Source: CAD feature listing. Evaluate the final solid. Frame: model axes, mm. Face numbers are marked on the shaded views. A direction names the side the tool comes from. Give positions to 0.01 mm unless a question says otherwise; leave off trailing zeros. Order: outer loops, then holes, each group sorted by start corner. A loop starts at its lowest first (then second) coordinate and runs counter-clockwise, first axis right, second up.
1) Section C-C, the plane x = -15. Return loops of the section in (y, z), plus the area to 3 significant figures.
2) Section A-A, the plane y = 4.75. Return loops of the section in (x, z) (1 decimal).
3) Section B-B, the plane z = -11.07. Return loops of the section in (x, y) (3 decimals), plus the area to 3 significant figures.
4) Material intervals for line 1 (X direction, y = 2.25, z = 2.75) (1 decimal); line 2 (Z direction, x = -26, y = 2.25); line 3 (Y direction, x = 9.5, z = 6.25), sorted ascending.
5) Draft query along X for the marked faces 4, 5 and 6. Return one class per face: released by +X, released by -X, zero draft, split by the parting line, or undercut.
6) Access query for the marked faces 1, 2 and 3. Directions: +Z, -Z, +X, -X, +Y, -Y. A direction counts if a zero-diameter tool reaches every point of the face in a straight line with its end or side. Return the directions, or none.
7) Section D-D, the plane z = 6.5. Return loops of the section in (x, y) (1 decimal), plus the area to 3 significant figures.
8) First-contact query: P1, Ø1.9, axis at x = -15.5, z = 5.5, coming from the +Y side; P2, Ø2, axis at y = 3, z = 5, coming from the -X side; P3, Ø2, axis at y = 3, z = 4.5, coming from the +X side (3 decimals); P4, Ø4, axis at x = 27, y = 7.5, coming from the -Z side. Flat tips, straight axial feed; report the tip coordinate or a pass-through.
Autodesk Inventor part; units mm, degrees
ref_plane "YZ Plane" through (0, 0, 0) normal (1, 0, 0) x (0, 1, 0)
ref_plane "XZ Plane" through (0, 0, 0) normal (0, 1, 0) x (-1, 0, 0)
ref_plane "XY Plane" through (0, 0, 0) normal (0, 0, 1) x (1, 0, 0)
sketch "Sketch1" plane through (0, 0, 0) normal (0, 1, 0) x (-1, 0, 0)
  line L0 (36.775, 13.07) -> (-36.775, 13.07)
  line L1 (-36.775, 13.07) -> (-36.775, -13.07)
  line L2 (-36.775, -13.07) -> (36.775, -13.07)
  line L3 (36.775, -13.07) -> (36.775, 13.07)
  line L4 (36.775, 13.07) -> (-36.775, -13.07) construction
  line L5 (-36.775, 13.07) -> (36.775, -13.07) construction
  circle A0 centre (-34.775, -11.07) radius 1.75
  circle A1 centre (34.775, 11.07) radius 1.75
  line L6 (-14.775, -0.61) -> (-24.775, -0.61)
  line L7 (-24.775, -0.61) -> (-24.775, 11.07)
  line L8 (-24.775, 11.07) -> (-14.775, 11.07)
  line L9 (-14.775, 11.07) -> (-14.775, -0.61)
  line L10 (-14.775, -0.61) -> (-24.775, 11.07) construction
  line L11 (-24.775, -0.61) -> (-14.775, 11.07) construction
  line L12 (28.4695, 2.1) -> (22.2095, 2.1)
  line L13 (22.2095, 2.1) -> (22.2095, 8.36)
  line L14 (22.2095, 8.36) -> (28.4695, 8.36)
  line L15 (28.4695, 8.36) -> (28.4695, 2.1)
  line L16 (28.4695, 2.1) -> (22.2095, 8.36) construction
  line L17 (22.2095, 2.1) -> (28.4695, 8.36) construction
  line L18 (18.4695, 8.36) -> (12.2095, 8.36)
  line L19 (12.2095, 8.36) -> (12.2095, 2.1)
  line L20 (12.2095, 2.1) -> (18.4695, 2.1)
  line L21 (18.4695, 2.1) -> (18.4695, 8.36)
  line L22 (18.4695, 8.36) -> (12.2095, 2.1) construction
  line L23 (12.2095, 8.36) -> (18.4695, 2.1) construction
  line L24 (8.4695, 8.36) -> (2.2095, 8.36)
  line L25 (2.2095, 8.36) -> (2.2095, 2.1)
  line L26 (2.2095, 2.1) -> (8.4695, 2.1)
  line L27 (8.4695, 2.1) -> (8.4695, 8.36)
  line L28 (8.4695, 8.36) -> (2.2095, 2.1) construction
  line L29 (2.2095, 8.36) -> (8.4695, 2.1) construction
  line L30 (-1.5305, 8.36) -> (-7.7905, 8.36)
  line L31 (-7.7905, 8.36) -> (-7.7905, 2.1)
  line L32 (-7.7905, 2.1) -> (-1.5305, 2.1)
  line L33 (-1.5305, 2.1) -> (-1.5305, 8.36)
  line L34 (-1.5305, 8.36) -> (-7.7905, 2.1) construction
  line L35 (-7.7905, 8.36) -> (-1.5305, 2.1) construction
  point P0 (0, 0)
  point P1 (-19.775, 5.23)
  point P2 (25.3395, 5.23)
  point P3 (15.3395, 5.23)
  point P4 (5.3395, 5.23)
  point P5 (-4.6605, 5.23)
  dimension "d0" = 73.55
  dimension "d1" = 26.14
  dimension "d2" = 3.5
  dimension "d3" = 2
  dimension "d4" = 2
  dimension "d5" = 3.5
  dimension "d6" = 2
  dimension "d7" = 2
  dimension "d8" = 10
  dimension "d9" = 11.68
  dimension "d10" = 12
  dimension "d11" = 2
  dimension "d12" = 6.26
  dimension "d13" = 6.26
  dimension "d14" = 6.26
  dimension "d15" = 6.26
  dimension "d16" = 10
  dimension "d17" = 6.26
  dimension "d18" = 6.26
  dimension "d19" = 10
  dimension "d20" = 6.26
  dimension "d21" = 6.26
  dimension "d22" = 10
  dimension "d23" = 6.9845
extrude "Extrusion1" add sketch "Sketch1" along normal blind 1.6
extrude "Extrusion2" add sketch "Sketch1" along normal blind 8.76 contours L6 L7 L8 L9
extrude "Extrusion3" add sketch "Sketch1" along normal blind 6 contours L12 L13 L14 L15 | L21 L20 L19 L18 | L27 L26 L25 L24 | L33 L32 L31 L30
sketch "Sketch2" plane through (0, 1.6, 0) normal (0, 1, 0) x (1, 0, 0)
  line L0 (-31.8499, 8.687) -> (29.6525, 8.687) construction
  line L1 (29.6525, 8.687) -> (29.6525, 4.9573) construction
  line L2 (29.6525, 4.9573) -> (-31.8499, 4.9573) construction
  line L3 (-31.8499, 4.9573) -> (-31.8499, 8.687) construction
  point P0 (0, 0)
properties part number "mode"
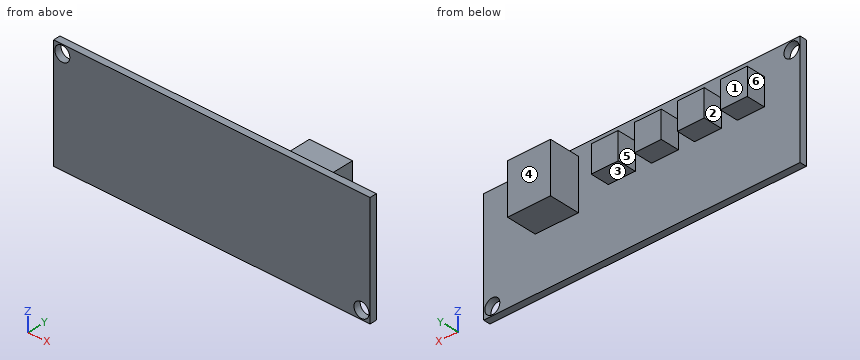
From the geometry:
1. outline: (0, -13.07) - (1.6, -13.07) - (1.6, 2.1) - (6, 2.1) - (6, 8.36) - (1.6, 8.36) - (1.6, 13.07) - (0, 13.07) - close
1. area: 69.4 mm2
2. outline: (-28.5, 2.1) - (-22.2, 2.1) - (-22.2, 8.4) - (-28.5, 8.4) - close; (-18.5, 2.1) - (-12.2, 2.1) - (-12.2, 8.4) - (-18.5, 8.4) - close; (-8.5, 2.1) - (-2.2, 2.1) - (-2.2, 8.4) - (-8.5, 8.4) - close; (1.5, 2.1) - (7.8, 2.1) - (7.8, 8.4) - (1.5, 8.4) - close; (14.8, -0.6) - (24.8, -0.6) - (24.8, 11.1) - (14.8, 11.1) - close
3. outline: (-36.775, 0) - (33.025, 0) - (33.025, 1.6) - (-36.775, 1.6) - close; (36.525, 0) - (36.775, 0) - (36.775, 1.6) - (36.525, 1.6) - close
3. area: 112 mm2
4. line 1: x = -28.5 to -22.2, -18.5 to -12.2, -8.5 to -2.2, 1.5 to 7.8, 14.8 to 24.8
4. line 2: z = 2.1 to 8.36
4. line 3: y = 0 to 1.6
5. face 4: zero draft
5. face 5: undercut
5. face 6: released by -X
6. face 1: +Z, -Z, -X, +Y
6. face 2: +Z, -Z, +Y
6. face 3: -Z, -X, +Y
7. outline: (-36.8, 0) - (36.8, 0) - (36.8, 1.6) - (24.8, 1.6) - (24.8, 8.8) - (14.8, 8.8) - (14.8, 1.6) - (7.8, 1.6) - (7.8, 6) - (1.5, 6) - (1.5, 1.6) - (-2.2, 1.6) - (-2.2, 6) - (-8.5, 6) - (-8.5, 1.6) - (-12.2, 1.6) - (-12.2, 6) - (-18.5, 6) - (-18.5, 1.6) - (-22.2, 1.6) - (-22.2, 6) - (-28.5, 6) - (-28.5, 1.6) - (-36.8, 1.6) - close
7. area: 299 mm2
8. P1: stops at y = 6
8. P2: stops at x = -28.47
8. P3: stops at x = 24.775
8. P4: passes through
